Input: part model. Units: mm. Frame: model coordinates. A direction names the side the tool comes from. Coordinates: 2 decimals unless noted, no trailing zeros. Order: outer loops, then holes, each group sorted by start corner. A loop starts at its lowest first (then second) coordinate and runs counter-clockwise, first axis right, second up. Notation, with made-up numbers: (-6.5, -21.75) - (40.5, -21.75) arc R15 ccw to (40.5, -17.75) - close; hole circle Ø8 at (77, 31.5). An arc over 180 degrees is marked (long way). One line per question, with ' | ' between items. Start each with the question number.
```python
from build123d import *

# Parameters (mm, degrees)
BOSS_EXTRUDE3_DEPTH       = 22.86
BOSS_EXTRUDE4_DEPTH       = 2.54
FILLET1_R                 = 2.54
SKETCH4_W                 = 8.004359919
SKETCH4_H                 = 7.259840527
CUT_EXTRUDE1_DEPTH        = 32.004
CUT_EXTRUDE1_DEPTH_BACK   = 2.54
F_8_CLEARANCE_HOLE1_D     = 4.3053
F_8_CLEARANCE_HOLE1_DEPTH = 74.422
F_8_CLEARANCE_HOLE1_TIP   = 1.293442612
F_8_CLEARANCE_HOLE2_D     = 4.3053
F_8_CLEARANCE_HOLE2_DEPTH = 74.422
F_8_CLEARANCE_HOLE2_TIP   = 1.293442612
F_8_CLEARANCE_HOLE3_D     = 4.3053
F_8_CLEARANCE_HOLE3_DEPTH = 74.422
F_8_CLEARANCE_HOLE3_TIP   = 1.293442612
FILLET2_R                 = 2.54
SKETCH11_R                = 2.159
CUT_EXTRUDE2_DEPTH        = 7.62
SKETCH12_R                = 2.159
CUT_EXTRUDE3_DEPTH        = 7.62


with BuildPart() as part:
    # Sketch1 → Boss-Extrude3 (new body)
    with BuildSketch(Plane(origin=(0, 0, 0), x_dir=(1, 0, 0), z_dir=(0, 1, 0))):
        Polygon((102.616, 2.54), (102.616, 0), (0, 0), (0, 102.616), (2.54, 102.616), (2.54, 2.54), align=None)
    extrude(amount=BOSS_EXTRUDE3_DEPTH)

    # Sketch3 → Boss-Extrude4 (add)
    with BuildSketch(Plane(origin=(0, 22.86, 0), x_dir=(1, 0, 0), z_dir=(0, 1, 0))):
        Polygon((2.54, 102.616), (102.616, 2.54), (2.54, 2.54), align=None)
    extrude(amount=-BOSS_EXTRUDE4_DEPTH)

    # Fillet1
    fillet1_edges = [part.edges().sort_by_distance(p)[0] for p in [
        (0, 22.86, -51.308),
        (51.308, 22.86, 0),
        (2.54, 10.16, -2.54),
        (52.578, 20.32, -2.54),
        (2.54, 20.32, -52.578),
    ]]
    fillet(fillet1_edges, radius=FILLET1_R)

    # Sketch4 → Cut-Extrude1 (cut, two sides)
    with BuildSketch(Plane.XZ.offset(-20.32)) as cut_extrude1_sk:
        with Locations((1.077820041, -1.450079736)):
            Rectangle(SKETCH4_W, SKETCH4_H)
    extrude(amount=CUT_EXTRUDE1_DEPTH, mode=Mode.SUBTRACT)
    extrude(cut_extrude1_sk.sketch, amount=-CUT_EXTRUDE1_DEPTH_BACK, mode=Mode.SUBTRACT)

    # #8 Clearance Hole1
    with Locations(Plane(origin=(2.54, 0, 0), x_dir=(0, 0, -1), z_dir=(1, 0, 0))):
        with Locations((39.116, 8.73125), (89.916, 8.73125)):
            Hole(F_8_CLEARANCE_HOLE1_D / 2, depth=F_8_CLEARANCE_HOLE1_DEPTH)
            with Locations((0, 0, -(F_8_CLEARANCE_HOLE1_DEPTH + F_8_CLEARANCE_HOLE1_TIP / 2))):  # 118° drill point
                Cone(0, F_8_CLEARANCE_HOLE1_D / 2, F_8_CLEARANCE_HOLE1_TIP, mode=Mode.SUBTRACT)

    # #8 Clearance Hole2
    with Locations(Plane.XY):
        with Locations((89.916, 8.73125), (39.116, 8.73125)):
            Hole(F_8_CLEARANCE_HOLE2_D / 2, depth=F_8_CLEARANCE_HOLE2_DEPTH)
            with Locations((0, 0, -(F_8_CLEARANCE_HOLE2_DEPTH + F_8_CLEARANCE_HOLE2_TIP / 2))):  # 118° drill point
                Cone(0, F_8_CLEARANCE_HOLE2_D / 2, F_8_CLEARANCE_HOLE2_TIP, mode=Mode.SUBTRACT)

    # #8 Clearance Hole3
    with Locations(Plane(origin=(0, 20.32, 0), x_dir=(-1, 0, 0), z_dir=(0, -1, 0))):
        with Locations((-16.010384182, 71.185103576), (-71.185103576, 16.010384182)):
            Hole(F_8_CLEARANCE_HOLE3_D / 2, depth=F_8_CLEARANCE_HOLE3_DEPTH)
            with Locations((0, 0, -(F_8_CLEARANCE_HOLE3_DEPTH + F_8_CLEARANCE_HOLE3_TIP / 2))):  # 118° drill point
                Cone(0, F_8_CLEARANCE_HOLE3_D / 2, F_8_CLEARANCE_HOLE3_TIP, mode=Mode.SUBTRACT)

    # Fillet2
    fillet2_edges = [part.edges().sort_by_distance(p)[0] for p in [
        (1.27, 0, -5.08),
        (5.08, 0, -1.27),
        (1.27, 0, -102.616),
        (102.616, 0, -1.27),
    ]]
    fillet(fillet2_edges, radius=FILLET2_R)

    # Sketch11 → Cut-Extrude2 (cut)
    with BuildSketch(Plane(origin=(2.54, 0, 0), x_dir=(0, 0, -1), z_dir=(1, 0, 0))):
        with Locations((79.0575, 8.73125)):
            Circle(SKETCH11_R)
    extrude(amount=-CUT_EXTRUDE2_DEPTH, mode=Mode.SUBTRACT)

    # Sketch12 → Cut-Extrude3 (cut)
    with BuildSketch(Plane.XY):
        with Locations((79.0575, 8.73125)):
            Circle(SKETCH12_R)
    extrude(amount=-CUT_EXTRUDE3_DEPTH, mode=Mode.SUBTRACT)


solid = part.part
```
(1) Reachability of faces 1 (the face through (32, 20.32, -32)), 2 (the face through (0, 10, -53)), 3 (the face through (53, 9, -2.54)) from +Z, -Z, +X, -X, +Y, -Y: full face, straight path, thin tool, end or side. Return the list, or none.
(2) Section C-C (z = -32.5). Output: boundary loops of the cut face in (x, y), then the cut area to 3 significant figures.
(3) Section D-D (x = 45). Output: boundary loops of the cut face in (y, z).
(4) Section B-B (x = 16). Output: boundary loops of the cut face in (y, z).
(5) Material intervals for line 1 along Y through (x, z) = (36, -57); line 2 along X through (y, z) = (17, -18); line 3 along Z through (x, y) = (86, 3), sorted ascending. Write a range as from..to.
(6) Section A-A (y = 13.5). Output: boundary loops of the cut face in (x, z).
(7) Pin query (flat end, axial travel): pin 1 (7 mm diameter, centred on y = 8.73, z = -89.92, fed in from -X); pin 2 (5 mm diameter, centred on y = 8.73, z = -39.12, fed in from +X); pin 3 (2 mm diameter, centred on x = 86, y = 13.5, fed in from -Z); pin 4 (3.5 mm diameter, centred on x = 39.12, y = 8.73, fed in from -Z). Return the tip coordinate at first contact, or that it passes through.
(8) Draft query along X for faces 4 (the face through (76.9, 8.8, -1.3)), 5 (the face through (3.304, 19.596, -54.531)), 6 (the face through (5.08, 15, -1)), 7 (the face through (31, 22.86, -31)). Return one class per face: +X half, -X half, draft (parallel to the pull), parting line (faces both ways), or undercut.
Worked answers:
1) face 1: -Z, +X, -Y | face 2: +Z, -Z, -X, +Y, -Y | face 3: -Z, +X, -X, -Y
2) outline: (0, 0) - (2.54, 0) - (2.54, 17.78) arc R2.54 cw to (5.08, 20.32) - (72.66, 20.32) - (72.66, 22.86) - (2.54, 22.86) arc R2.54 ccw to (0, 20.32) - close | area: 236 mm²
3) outline: (0, -2.54) - (17.78, -2.54) arc R2.54 cw to (20.32, -5.08) - (20.32, -60.16) - (22.86, -60.16) - (22.86, -2.54) arc R2.54 ccw to (20.32, 0) - (0, 0) - close
4) outline: (0, -2.54) - (17.78, -2.54) arc R2.54 cw to (20.32, -5.08) - (20.32, -69.03) - (22.86, -69.03) - (22.86, -2.54) arc R2.54 ccw to (20.32, 0) - (0, 0) - close; (20.32, -89.16) - (22.86, -89.16) - (22.86, -73.34) - (20.32, -73.34) - close
5) line 1: y = 20.32..22.86 | line 2: x = 0..2.54 | line 3: z = -2.54..0
6) outline: (0, -102.62) - (2.54, -102.62) - (2.54, -5.08) - (0, -5.08) - close; (5.08, -2.54) - (102.62, -2.54) - (102.62, 0) - (5.08, 0) - close
7) pin 1: stops at x = 0 | pin 2: stops at x = 2.54 | pin 3: stops at z = -2.54 | pin 4: passes through
8) face 4: undercut | face 5: +X half | face 6: -X half | face 7: draft
